Work out the finished part from the listing and answer in its coordinate system (mm). Face numbers are marked on the shaded views. Coordinates: 2 decimals unless noted, no trailing zeros. Write each loop counter-clockwise with the first axis right and the second up, starting at its lowest first coordinate (ties: lowest second). Pieces come first, ordered by that corner, then holes. Notation, with made-up numbers: M 41.5,31.5 L 99.5,31.5 A11 cw 99.5,49.5 Z; hole C 53,80.5 d11. An arc over 180 degrees is marked long. Answer as CSV lines item,"result". Start each with the question number.
(1) A cutting plane is placed at C-C on x = 15. Give the vertices of the cut face in (y, z) (3 decimals).
(2) A cutting plane is placed at A-A on z = 0. Give the vertices of the cut face in (x, y) (3 decimals).
(3) The mould has two halves that part along Z. Classify the marked faces 1, 2, 3 and 4: released by +Z, released by -Z, zero draft, split by the parting line, or undercut.
(4) A cutting plane is placed at D-D on z = 16.25. Give the vertices of the cut face in (x, y) (3 decimals).
(5) Find the intervals of material crossed by L1, parallel to Z at x = 20.5, y = 2.05 (3 decimals); L2, parallel to X at y = 1.9, z = 0 (3 decimals); L3, parallel to Z at x = 1, y = 1.75 (3 decimals), in increasing order. Write a range as [from, to].
(6) Flat-ended cylindrical pins translate along their axes: P1, Ø1, axis at x = 5.5, y = 2, coming from the +Z side (3 decimals); P2, Ø1, axis at y = 1, z = 15, coming from the -X side. Find the tip coordinate at first contact, or state that the pin passes through.
(7) A cutting plane is placed at B-B on y = 2.7. Give the vertices of the cut face in (x, z) (3 decimals), then the cut area to 3 significant figures.
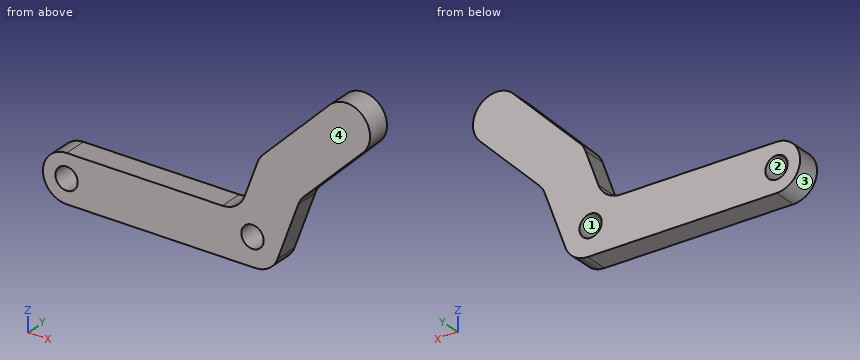
from build123d import *

# Parameters (mm, degrees)
SKETCH1_R           = 1.5
BOSS_EXTRUDE1_DEPTH = 3.175


with BuildPart() as part:
    # Sketch1 → Boss-Extrude1 (new body)
    with BuildSketch(Plane(origin=(0, 0, 0), x_dir=(1, 0, 0), z_dir=(0, 1, 0))):
        with BuildLine():
            Line((0, -3.175), (20.953682132, -3.175))
            ThreePointArc((20.953682132, -3.175), (22.774787318, -3.749192259), (23.937206203, -5.264086045))
            Line((23.937206203, -5.264086045), (25.674217794, -10.036486168))
            ThreePointArc((25.674217794, -10.036486168), (25.979974025, -10.656498469), (26.412677835, -11.195636243))
            Line((26.412677835, -11.195636243), (35.392933956, -20.175892364))
            ThreePointArc((35.392933956, -20.175892364), (39.883062017, -20.175892364), (39.883062017, -15.685764304))
            Line((39.883062017, -15.685764304), (31.898243321, -7.700945608))
            ThreePointArc((31.898243321, -7.700945608), (31.465539511, -7.161807835), (31.15978328, -6.541795533))
            Line((31.15978328, -6.541795533), (28.383524071, 1.085913955))
            ThreePointArc((28.383524071, 1.085913955), (27.221105185, 2.600807741), (25.4, 3.175))
            Line((25.4, 3.175), (0, 3.175))
            ThreePointArc((0, 3.175), (-3.175, 0), (0, -3.175))
        make_face()
        with Locations(Location((24.997946252, -0.574192259, 0), (0, 0, 270))):
            Circle(SKETCH1_R, mode=Mode.SUBTRACT)
        with Locations(Location((0, 0, 0), (0, 0, 270))):
            Circle(SKETCH1_R, mode=Mode.SUBTRACT)
    extrude(amount=BOSS_EXTRUDE1_DEPTH)


solid = part.part
Here are the results:
1,outline,"M 0,-3.175 L 3.175,-3.175 L 3.175,3.175 L 0,3.175 Z"
2,outline,"M -3.175,0 L -1.5,0 L -1.5,3.175 L -3.175,3.175 Z; M 1.5,0 L 23.612,0 L 23.612,3.175 L 1.5,3.175 Z; M 26.384,0 L 28.779,0 L 28.779,3.175 L 26.384,3.175 Z"
3,face 1,"undercut"
3,face 2,"undercut"
3,face 3,"split by the parting line"
3,face 4,"zero draft"
4,outline,"M 31.467,0 L 40.332,0 L 40.332,3.175 L 31.467,3.175 Z"
5,L1,"z = [-3.175, 3.175]"
5,L2,"x = [-3.175, -1.5], [1.5, 23.612], [26.384, 28.779]"
5,L3,"z = [-3.175, -1.118], [1.118, 3.175]"
6,P1,"stops at z = 3.175"
6,P2,"stops at x = 29.72"
7,outline,"M 0,-3.175 L 25.4,-3.175 A3.175 ccw 28.384,-1.086 L 31.16,6.542 A3.175 cw 31.898,7.701 L 39.883,15.686 A3.175 ccw 35.393,20.176 L 26.413,11.196 A3.175 ccw 25.674,10.036 L 23.937,5.264 A3.175 cw 20.954,3.175 L 0,3.175 A3.175 ccw Z; hole C 0,0 d3; hole C 24.998,0.574 d3"
7,area,"320 mm^2"
